```python
from build123d import *

# Parameters (mm, degrees)
BOSS_EXTRUDE1_DEPTH = 6.35
SKETCH2_R           = 6.985
SKETCH2_W           = 5.334
SKETCH2_H           = 1.778
CUT_EXTRUDE1_DEPTH  = 10.16
SKETCH3_W           = 1.778
SKETCH3_H           = 5.334
CUT_EXTRUDE2_DEPTH  = 10.16
SKETCH4_R           = 1.1303
CUT_EXTRUDE3_DEPTH  = 10.16
SKETCH5_W           = 17.78
SKETCH5_H           = 19.05
SKETCH5_H_2         = 18.9992
CUT_EXTRUDE4_DEPTH  = 10.16


with BuildPart() as part:
    # Sketch1 → Boss-Extrude1 (new body)
    with BuildSketch(Plane(origin=(0, 0, 0), x_dir=(1, 0, 0), z_dir=(0, 1, 0))):
        Polygon((-95.504, 15.875), (-101.6, 15.875), (-101.6, -15.875), (-95.504, -15.875), (-95.504, -33.02), (-70.104, -33.02), (-70.104, -19.812), (-63.5, -19.812), (-63.5, -33.02), (2.794, -33.02), (9.398, -33.02), (62.484, -33.02), (62.484, -19.812), (69.088, -19.812), (69.088, -33.02), (94.488, -33.02), (94.488, -15.875), (100.584, -15.875), (100.584, 15.875), (94.488, 15.875), (94.488, 33.02), (69.088, 33.02), (69.088, 19.812), (62.484, 19.812), (62.484, 33.02), (9.398, 33.02), (2.794, 33.02), (-63.5, 33.02), (-63.5, 19.812), (-70.104, 19.812), (-70.104, 33.02), (-95.504, 33.02), align=None)
    extrude(amount=BOSS_EXTRUDE1_DEPTH)

    # Sketch2 → Cut-Extrude1 (cut)
    with BuildSketch(Plane(origin=(0, 6.35, 0), x_dir=(1, 0, 0), z_dir=(0, 1, 0))):
        with Locations(Location((18.796, 17.78, 0), (0, 0, 270))):
            Circle(SKETCH2_R)
        with Locations((-47.371, 16.764)):
            Rectangle(SKETCH2_W, SKETCH2_H)
        with Locations((-47.371, -16.764)):
            Rectangle(SKETCH2_W, SKETCH2_H)
        with Locations((47.879, 16.764)):
            Rectangle(SKETCH2_W, SKETCH2_H)
        with Locations((47.879, -16.764)):
            Rectangle(SKETCH2_W, SKETCH2_H)
    extrude(amount=-CUT_EXTRUDE1_DEPTH, mode=Mode.SUBTRACT)

    # Sketch3 → Cut-Extrude2 (cut)
    with BuildSketch(Plane(origin=(0, 6.35, 0), x_dir=(1, 0, 0), z_dir=(0, 1, 0))):
        with Locations((-75.565, 0)):
            Rectangle(SKETCH3_W, SKETCH3_H)
        with Locations((-15.367, 0)):
            Rectangle(SKETCH3_W, SKETCH3_H)
        with Locations((14.351, 0)):
            Rectangle(SKETCH3_W, SKETCH3_H)
        with Locations((74.549, 0)):
            Rectangle(SKETCH3_W, SKETCH3_H)
    extrude(amount=-CUT_EXTRUDE2_DEPTH, mode=Mode.SUBTRACT)

    # Sketch4 → Cut-Extrude3 (cut)
    with BuildSketch(Plane(origin=(0, 6.35, 0), x_dir=(1, 0, 0), z_dir=(0, 1, 0))):
        with Locations(Location((-38.1, 26.67, 0), (0, 0, 270))):
            Circle(SKETCH4_R)
        with Locations(Location((37.084, 26.67, 0), (0, 0, 270))):
            Circle(SKETCH4_R)
        with Locations(Location((-38.1, -26.67, 0), (0, 0, 270))):
            Circle(SKETCH4_R)
        with Locations(Location((37.084, -26.67, 0), (0, 0, 270))):
            Circle(SKETCH4_R)
    extrude(amount=-CUT_EXTRUDE3_DEPTH, mode=Mode.SUBTRACT)

    # Sketch5 → Cut-Extrude4 (cut)
    with BuildSketch(Plane.XZ):
        with Locations((-92.71, 0)):
            Rectangle(SKETCH5_W, SKETCH5_H)
        with Locations((91.694, -0.0254)):
            Rectangle(SKETCH5_W, SKETCH5_H_2)
    extrude(amount=-CUT_EXTRUDE4_DEPTH, mode=Mode.SUBTRACT)


solid = part.part
```
For this review, take the finished solid that the model builds, in its own axes (mm). A direction names the side the tool comes from. Round coordinates to 2 decimals unless told otherwise and drop trailing zeros. Write each loop counter-clockwise with the first axis right and the second up, starting at its lowest first coordinate (ties: lowest second). Pieces come first, ordered by that corner, then holes.
1) For line 1 along Z through (x, y) = (48, 5) (3 decimals); line 2 along X through (y, z) = (3.25, -26.67); line 3 along Z through (x, y) = (89.5, 1.25) (3 decimals), list the stretches that pass through material, from the lowest coordinate up.
Answer below:
line 1: z = -33.02 to -17.653, -15.875 to 15.875, 17.653 to 33.02
line 2: x = -95.5 to -70.1, -63.5 to -39.23, -36.97 to 35.95, 38.21 to 62.48, 69.09 to 94.49
line 3: z = -33.02 to -9.525, 9.474 to 33.02
2) Insertion check: pin 1 Ø1.9 at (y, z) = (4.5, -26.5) entering from -X; pin 2 Ø3 at (y, z) = (1, -1.5) entering from -X. Each pin has a flat end and moves straight along its axis. Give the tip position at first contact, or say it passes through.
Answer below:
pin 1: stops at x = -95.5
pin 2: stops at x = -83.82
3) Take a section at A-A on z = 22.5. Give the boundary of the cut face in (x, y).
Answer below:
outline: (-95.5, 0) - (-70.1, 0) - (-70.1, 6.35) - (-95.5, 6.35) - close; (-63.5, 0) - (62.48, 0) - (62.48, 6.35) - (-63.5, 6.35) - close; (69.09, 0) - (94.49, 0) - (94.49, 6.35) - (69.09, 6.35) - close
4) Take a section at C-C on y = 4.5. State how many separate pieces and enclosed holes the cut face has, then the cut area to 3 significant figures.
Answer below:
separate pieces: 1
enclosed holes: 13
area: 11,700 mm2
5) Machinability: for faces 4 (the face through (-76.454, 3, 0)), 5 (the face through (-67, 3, 19.812)), 6 (the face through (92, 3, -9.525)), 7 (the face through (-70.104, 3, -26)), 8 (the face through (-99, 3, 15.875)), which of the approach directions +Z, -Z, +X, -X, +Y, -Y give a long, thin tool a straight path to every point of the face, cutting with its end or side? Answer none if there is none.
Answer below:
face 4: +Y, -Y
face 5: +Z, +Y, -Y
face 6: +X, +Y, -Y
face 7: -Z, +Y, -Y
face 8: +Z, -X, +Y, -Y
6) Take a section at B-B on z = -12.5. Give the boundary of the cut face in (x, y).
Answer below:
outline: (-101.6, 0) - (14.22, 0) - (14.22, 6.35) - (-101.6, 6.35) - close; (23.37, 0) - (100.58, 0) - (100.58, 6.35) - (23.37, 6.35) - close
7) Mouldability with a two-part tool opening along X and no side actions: class faces 1 (the face through (-2, 0, 0)), 2 (the face through (-95.504, 3, 24)), 3 (the face through (66, 3, -19.812)) as +X half, -X half, draft (parallel to the pull), parting line (faces both ways), or undercut.
Answer below:
face 1: draft
face 2: -X half
face 3: undercut
